Design review of the part built by this model. Coordinates are the model's own, in mm. A direction names the side the tool comes from. Coordinates: 2 decimals unless noted, no trailing zeros. Loops run counter-clockwise (first coordinate to the right, second up) from the corner with the lowest first, then second, coordinate; pieces in that order, holes last. Notation, with made-up numbers: (88, 64) - (104, 64) arc R17 cw to (104, 87) - close; hole circle Ø1 at (21.25, 39). An arc over 180 degrees is marked (long way). One line per question, with ' | ' between items.
from build123d import *
from build123d.topology import SkipClean

# Parameters (mm, degrees)
EXTRUDE_1_DEPTH     = 25
EXTRUDE_START       = -3
EXTRUDE_2_DEPTH     = 3
EXTRUDE_START_2     = 22
SKETCH_3_R          = 1.649999999999988
SKETCH_3_R_2        = 1.6500000000000072
EXTRUDE_3_DEPTH     = 22
SKETCH_4_R          = 1.6499999999999844
SKETCH_4_R_2        = 1.6500000000000101
SKETCH_4_R_3        = 1.6499999999999744
CUT_EXTRUDE_1_DEPTH = 177.47813778434883
FILLET_1_R          = 10
SKETCH_7_R          = 1.9845527955415248
CUT_EXTRUDE_2_DEPTH = 177.0782017054684


with BuildPart() as part:
    # 草图1 → 凸台-拉伸1 (new body)
    with BuildSketch(Plane.XY):
        with BuildLine():
            ThreePointArc((-6.39904e-12, -143.5), (32.28047629834163, -139.82210429668194), (62.90625956423284, -128.97694564393035))
            Line((62.90625956423282, -128.97694564393035), (60.71440383028742, -124.48297541243448))
            ThreePointArc((60.71440383028932, -124.4829754124336), (31.15572102662481, -134.95025397275518), (-3.22377e-12, -138.5))
            Line((0, -138.49999999999997), (0, -143.49999999999997))
        make_face()
        with BuildLine():
            Line((-60.71440383028735, -124.48297541243457), (-62.906259564232734, -128.97694564393038))
            ThreePointArc((-62.906259564232776, -128.97694564393038), (-32.28047629834789, -139.8221042966805), (-6.39904e-12, -143.5))
            Line((0, -143.49999999999997), (0, -138.49999999999997))
            ThreePointArc((-3.22377e-12, -138.5), (-31.155721026627976, -134.95025397275447), (-60.71440383028926, -124.48297541243363))
        make_face()
    extrude(amount=EXTRUDE_1_DEPTH)

    # 草图2 → 凸台-拉伸2 (add)
    with BuildSketch(Plane.XY.offset(25).offset(EXTRUDE_START)):
        with BuildLine():
            Line((70.13938348625264, -143.8070474078666), (62.906259564232826, -128.97694564393032))
            ThreePointArc((62.90625956423283, -128.97694564393032), (4.796e-14, -143.5), (-62.90625956423274, -128.97694564393038))
            Line((-62.90625956423273, -128.97694564393043), (-70.13938348625253, -143.8070474078667))
            ThreePointArc((-70.13938348625257, -143.80704740786663), (-2.939e-14, -160), (70.13938348625264, -143.8070474078666))
        make_face()
    extrude(amount=EXTRUDE_2_DEPTH)

    # 草图3 → 凸台-拉伸3 (add)
    with SkipClean():  # the faces are left unmerged after this step: merging them gives an invalid solid
        with BuildSketch(Plane(origin=(0, 0, 22.000000000000004), x_dir=(-1, 0, 0), z_dir=(0, 0, -1)).offset(EXTRUDE_START_2)):
            with Locations(Location((-27.51756434931431, -148.4714910421571, 0), (0, 0, 180))):
                Circle(SKETCH_3_R)
            with Locations(Location((1.91e-14, -156, 0), (0, 0, 180))):
                Circle(SKETCH_3_R_2)
            with BuildLine():
                Line((-16.16900754927144, -159.18091341260617), (-14.501578645752826, -142.76538171693122))
                ThreePointArc((-14.501578645754455, -142.76538171693085), (-17.239636372772704, -142.46067856687523), (-19.971339987769433, -142.10346786441525))
                Line((-19.971339987769415, -142.10346786441528), (-22.267696153610498, -158.4428909986512))
                ThreePointArc((-22.26769615360823, -158.44289099865154), (-19.221894213540633, -158.84117470871163), (-16.169007549267842, -159.1809134126065))
            make_face()
            with BuildLine():
                ThreePointArc((19.9713399877666, -142.10346786441565), (17.239636372771262, -142.4606785668754), (14.501578645754403, -142.76538171693088))
                Line((14.50157864575282, -142.76538171693116), (16.16900754927144, -159.18091341260617))
                ThreePointArc((16.16900754926785, -159.1809134126065), (19.22189421354061, -158.84117470871166), (22.26769615360823, -158.44289099865156))
                Line((22.267696153610498, -158.4428909986512), (19.971339987769422, -142.10346786441534))
            make_face()
            with Locations((27.51756434931431, -148.4714910421571)):
                Circle(SKETCH_3_R)
        extrude(amount=-EXTRUDE_3_DEPTH)

    # 草图4 → 切除-拉伸1 (cut, through all)
    with SkipClean():  # the faces are left unmerged after this step: merging them gives an invalid solid
        with BuildSketch(Plane(origin=(0, 0, 0), x_dir=(-1, 0, 0), z_dir=(0, 0, -1))):
            with Locations((-27.51756434931431, -148.4714910421571)):
                Circle(SKETCH_4_R)
            with Locations((1.91e-14, -156)):
                Circle(SKETCH_4_R_2)
            with Locations((27.51756434931431, -148.4714910421571)):
                Circle(SKETCH_4_R_3)
        extrude(amount=-CUT_EXTRUDE_1_DEPTH, mode=Mode.SUBTRACT)

    # 草图6 → 切除-旋转1 (revolve, cut)
    with BuildSketch(Plane(origin=(0, 0, 0), x_dir=(0, 0, -1), z_dir=(0.9902680687415703, 0.13917310096006566, 0))):
        Polygon((6.94e-15, -143.5), (-22.000000000000007, -160), (6.94e-15, -160), align=None)
    revolve(axis=Axis((0, 0, 25), (0, 0, -1)), mode=Mode.SUBTRACT)

    # 圆角1
    fillet_1_edges = [part.edges().sort_by_distance(p)[0] for p in [
        (60.71440383028837, -124.48297541243404, 12.5),
        (-60.714403830288305, -124.48297541243412, 12.5),
    ]]
    fillet(fillet_1_edges, radius=FILLET_1_R)

    # 草图7 → 切除-拉伸2 (cut, through all)
    with BuildSketch(Plane(origin=(0, 0, 22.000000000000004), x_dir=(-1, 0, 0), z_dir=(0, 0, -1))):
        with Locations((50.73693085640144, -143.81242591401045)):
            Circle(SKETCH_7_R)
        with Locations(Location((-50.7369308564015, -143.81242591401042, 0), (0, 0, 180))):
            Circle(SKETCH_7_R)
    extrude(amount=-CUT_EXTRUDE_2_DEPTH, mode=Mode.SUBTRACT)


solid = part.part
Q1. To check wall thickness, follow line 1 along Z through (x, y) = (28.5, -157); line 2 along X through (y, z) = (-149, 10.25); line 3 along X through (y, z) = (-156, 20). State the ranges of each line that lie inside material, in increasing order.
Returned:
line 1: z = 22 to 25 | line 2: x = -20.94 to -15.13, 15.13 to 20.94 | line 3: x = -21.92 to -15.85, 15.85 to 21.92
Q2. Draft analysis for pull direction Y (two halves, no side actions). For faces 1 (the conical face through (18.285, -150.761, 11.154)), 2 (the cylindrical face through (27.88, -150.08, 23.48)), 3 (the flat face through (67.6, -138.6, 23.5)), state which applies: +Y half, -Y half, draft (parallel to the pull), parting line (faces both ways), or undercut.
Returned:
face 1: -Y half | face 2: undercut | face 3: +Y half
Q3. Take a section at B-B (z = 18). Give the boundary of the cut face in (x, y).
Returned:
outline: (-61.87, -129.48) arc R143.5 ccw to (-19.97, -142.1) - (-21.85, -155.47) arc R157 ccw to (-15.87, -156.2) - (-14.5, -142.77) arc R143.5 ccw to (14.5, -142.77) - (15.87, -156.2) arc R157 ccw to (21.85, -155.47) - (19.97, -142.1) arc R143.5 ccw to (61.87, -129.48) arc R10 ccw to (52.19, -128.29) arc R138.5 cw to (-52.19, -128.29) arc R10 ccw to start
Q4. Take a section at C-C (y = -140). Give the boundary of the cut face in (x, z).
Returned:
outline: (-68.28, 22) - (-31.5, 22) - (-31.5, 0) - (31.5, 0) - (31.5, 22) - (68.28, 22) - (68.28, 25) - (-68.28, 25) - close
Q5. For pin 1 (8 mm diameter, centred on x = -22, z = 6, fed in from +Y); pin 2 (5.5 mm diameter, centred on x = 0, y = -156, fed in from -Z); pin 3 (3 mm diameter, centred on x = 50.5, z = 20, fed in from -Y); pin 4 (3 mm diameter, centred on x = 50.74, y = -143.81, fed in from -Z), all flat-tipped, find the tip position at first contact; note any pin that passes through.
Returned:
pin 1: stops at y = -136.04 | pin 2: stops at z = 22 | pin 3: stops at y = -134.87 | pin 4: passes through
Q6. Take a section at A-A (x = 0). Give the boundary of the cut face in (y, z), plus the area to 3 significant figures.
Returned:
outline: (-160, 22) - (-157.65, 22) - (-157.65, 25) - (-160, 25) - close; (-154.35, 22) - (-143.5, 22) - (-143.5, 0) - (-138.5, 0) - (-138.5, 25) - (-154.35, 25) - close | area: 165 mm²
Q7. Take a section at D-D (x = -57). Give the boundary of the cut face in (y, z).
Returned:
outline: (-149.5, 22) - (-131.69, 22) - (-131.69, 0) - (-127.61, 0) - (-127.61, 25) - (-149.5, 25) - close
Q8. Tool access review of faces 4 (the flat face through (0, -151, 22)), 5 (the flat face through (-20.625, -146.757, 15.735)), 6 (the flat face through (0, -139, 0)): name each direction out of +Z, -Z, +X, -X, +Y, -Y from which nothing blocks a thin tool from reaching the whole face with its end or side.
Returned:
face 4: -Z, -Y | face 5: -Z, -X | face 6: -Z, +X, -X, +Y, -Y
